Design review of the part built by this model. Coordinates are the model's own, in mm. Coordinates: 2 decimals unless noted, no trailing zeros. Order: outer loops, then holes, each group sorted by start corner. A loop starts at its lowest first (then second) coordinate and runs counter-clockwise, first axis right, second up. Notation, with made-up numbers: M -12,-25.5 L 23,-25.5 A21 ccw 23,-8.5 Z; hole C 23.25,56.25 d4. An arc over 180 degrees is marked long. Answer as a JSON object with one key per item and string values.
from build123d import *

# Parameters (mm, degrees)
F1_DEPTH = 25.4


with BuildPart() as f1:
    # F0 (on Top) → F1 (new body)
    with BuildSketch(Plane.XY):
        with BuildLine():
            Line((327.025, 107.95), (327.025, 165.1))
            Line((327.025, 165.1), (0, 165.1))
            Line((0, 165.1), (0, -165.1))
            Line((0, -165.1), (327.025, -165.1))
            Line((327.025, -165.1), (327.025, -107.95))
            ThreePointArc((327.025, -107.95), (314.325, -95.25), (327.025, -82.55))
            Line((327.025, -82.55), (327.025, -44.45))
            ThreePointArc((327.025, -44.45), (314.325, -31.75), (327.025, -19.05))
            Line((327.025, -19.05), (327.025, 19.05))
            ThreePointArc((327.025, 19.05), (314.325, 31.75), (327.025, 44.45))
            Line((327.025, 44.45), (327.025, 82.55))
            ThreePointArc((327.025, 82.55), (314.325, 95.25), (327.025, 107.95))
        make_face()
        with BuildLine():
            Line((0, -165.1), (0, 165.1))
            Line((0, 165.1), (-327.025, 165.1))
            Line((-327.025, 165.1), (-327.025, 107.95))
            ThreePointArc((-327.025, 107.95), (-314.325, 95.25), (-327.025, 82.55))
            Line((-327.025, 82.55), (-327.025, 44.45))
            ThreePointArc((-327.025, 44.45), (-314.325, 31.75), (-327.025, 19.05))
            Line((-327.025, 19.05), (-327.025, -19.05))
            ThreePointArc((-327.025, -19.05), (-314.325, -31.75), (-327.025, -44.45))
            Line((-327.025, -44.45), (-327.025, -82.55))
            ThreePointArc((-327.025, -82.55), (-314.325, -95.25), (-327.025, -107.95))
            Line((-327.025, -107.95), (-327.025, -165.1))
            Line((-327.025, -165.1), (0, -165.1))
        make_face()
    extrude(amount=F1_DEPTH)


solid = f1.part
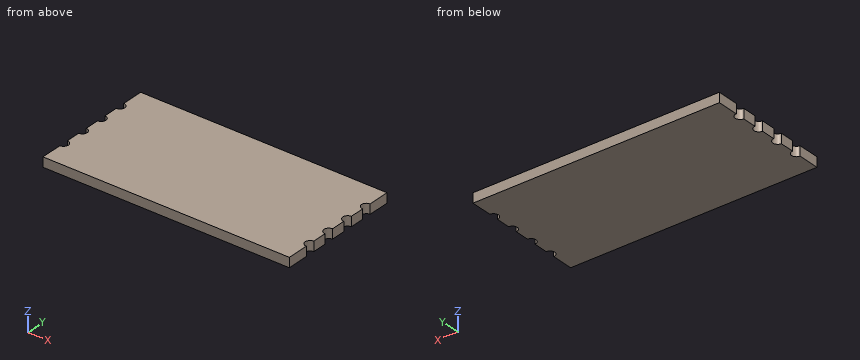
1) Add section B-B (y = 26.5). State the section outline as (x, z) points.
Taken from the geometry:
{"outline": "M -315.46,0 L 315.46,0 L 315.46,25.4 L -315.46,25.4 Z"}
2) Insertion check: pin 1 Ø1 at (y, z) = (-27.5, 3) entering from -X; pin 2 Ø4 at (y, z) = (36, 15) entering from +X. Each pin has a flat end and moves straight along its axis. Give the tip position at first contact, or say it passes through.
Taken from the geometry:
{"pin 1": "stops at x = -315.25", "pin 2": "stops at x = 315.97"}
3) Add section A-A (y = -95.25). State the section outline as (x, z) points (3 decimals), and give its area (3 significant figures).
Taken from the geometry:
{"outline": "M -314.325,0 L 314.325,0 L 314.325,25.4 L -314.325,25.4 Z", "area": "16,000 mm2"}
4) To check wall thickness, follow L1, parallel to X at y = -33.5, z = 12.25; L2, parallel to X at y = 88.5, z = 11. State the ranges of each line that lie inside material, in increasing order.
Taken from the geometry:
{"L1": "x = -314.45 to 314.45", "L2": "x = -316.27 to 316.27"}
